The model under review builds one solid part; all positions refer to its coordinate system, in mm. Face numbers are marked on the shaded views. A direction names the side the tool comes from. Give positions to 0.01 mm unless a question says otherwise; leave off trailing zeros. Order: outer loops, then holes, each group sorted by start corner. A loop starts at its lowest first (then second) coordinate and runs counter-clockwise, first axis right, second up.
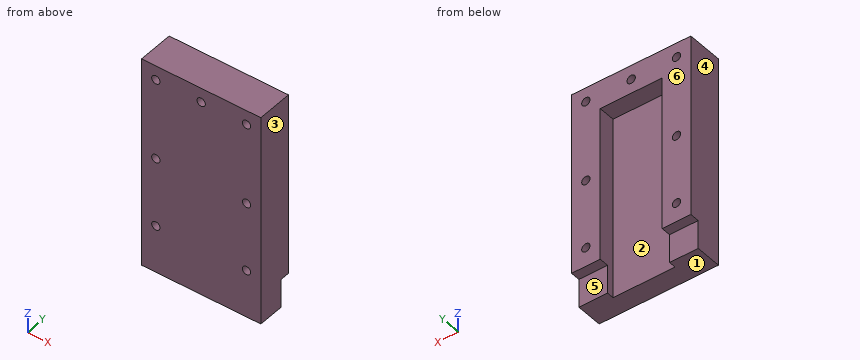
```python
from build123d import *

# Parameters (mm, degrees)
SKETCH_1_W          = 50
SKETCH_1_H          = 30
EXTRUDE_1_DEPTH     = 89
SKETCH_2_W          = 26
SKETCH_2_H          = 14
CUT_EXTRUDE_1_DEPTH = 77
SKETCH_5_W          = 12
SKETCH_5_H          = 8
CUT_EXTRUDE_4_DEPTH = 98.928545379
SKETCH_6_W          = 12
SKETCH_6_H          = 8
CUT_EXTRUDE_5_DEPTH = 98.928545379
SKETCH_7_R          = 1.75
CUT_EXTRUDE_6_DEPTH = 98.190534519


with BuildPart() as part:
    # ｽｹｯﾁ1 → ﾎﾞｽ - 押し出し1 (new body)
    with BuildSketch(Plane.XY):
        Rectangle(SKETCH_1_W, SKETCH_1_H)
    extrude(amount=EXTRUDE_1_DEPTH)

    # ｽｹｯﾁ2 → ｶｯﾄ - 押し出し1 (cut)
    with BuildSketch(Plane(origin=(0, 0, 0), x_dir=(-1, 0, 0), z_dir=(0, 0, -1))):
        Rectangle(SKETCH_2_W, SKETCH_2_H)
    extrude(amount=-CUT_EXTRUDE_1_DEPTH, mode=Mode.SUBTRACT)

    # ｽｹｯﾁ5 → ｶｯﾄ - 押し出し4 (cut, through all)
    with BuildSketch(Plane.ZY.offset(-13)):
        with Locations((6, 0)):
            Rectangle(SKETCH_5_W, SKETCH_5_H)
    extrude(amount=-CUT_EXTRUDE_4_DEPTH, mode=Mode.SUBTRACT)

    # ｽｹｯﾁ6 → ｶｯﾄ - 押し出し5 (cut, through all)
    with BuildSketch(Plane(origin=(-13, 0, 0), x_dir=(0, 0, -1), z_dir=(1, 0, 0))):
        with Locations((-6, 0)):
            Rectangle(SKETCH_6_W, SKETCH_6_H)
    extrude(amount=-CUT_EXTRUDE_5_DEPTH, mode=Mode.SUBTRACT)

    # ｽｹｯﾁ7 → ｶｯﾄ - 押し出し6 (cut, through all)
    with BuildSketch(Plane(origin=(0, 15, 0), x_dir=(1, 0, 0), z_dir=(0, 1, 0))):
        with Locations(Location((19, -20, 0), (0, 0, 270))):
            Circle(SKETCH_7_R)
        with Locations(Location((19, -49, 0), (0, 0, 270))):
            Circle(SKETCH_7_R)
        with Locations(Location((19, -83, 0), (0, 0, 270))):
            Circle(SKETCH_7_R)
        with Locations(Location((0, -83, 0), (0, 0, 270))):
            Circle(SKETCH_7_R)
        with Locations(Location((-19, -83, 0), (0, 0, 270))):
            Circle(SKETCH_7_R)
        with Locations(Location((-19, -49, 0), (0, 0, 270))):
            Circle(SKETCH_7_R)
        with Locations(Location((-19, -20, 0), (0, 0, 270))):
            Circle(SKETCH_7_R)
    extrude(amount=-CUT_EXTRUDE_6_DEPTH, mode=Mode.SUBTRACT)

    # Surface Cut 1
    split(bisect_by=Plane(origin=(0, 0, 0), x_dir=(-1, 0, 0), z_dir=(0, -1, 0)), keep=Keep.TOP)


solid = part.part
```
1. Take a section at C-C (z = 20). Write out the cut boundary in (x, y), and give its area (3 significant figures).
2. Take a section at D-D (z = 83). Write out the cut boundary in (x, y), and give its area (4 significant figures).
3. Insertion check: pin 1 (4 mm diameter, centred on x = 15.5, y = -5.5, fed in from -Z); pin 2 (3 mm diameter, centred on x = 18.5, y = -2, fed in from -Z); pin 3 (3.5 mm diameter, centred on x = -18.5, z = 4, fed in from +Y); pin 4 (3.5 mm diameter, centred on x = -4.5, y = -4.5, fed in from -Z). Each pin has a flat end and moves straight along its axis. Give the tip position at first contact, or say it passes through.
4. To check wall thickness, follow line 1 (X direction, y = -6, z = 49); line 2 (X direction, y = -12, z = 49); line 3 (X direction, y = -7, z = 83). State the ranges of each line that lie inside material, in increasing order.
5. Draft analysis for pull direction X (two halves, no side actions). For the marked faces 1, 2, 3 and 4, state which applies: pulls with the +X half, pulls with the -X half, needs draft (parallel to the pull), parting line crosses it, or undercut.
6. Take a section at B-B (y = -6). Write out the cut boundary in (x, z).
7. For the marked faces 5 and 6, list the 3-axis set-ups (+Z, -Z, +X, -X, +Y, -Y) from which the entire face can be reached by the end or side of a thin tool; tool diameter is ignored.
8. Take a section at A-A (x = 19). Write out the cut boundary in (y, z), and give its area (3 significant figures).
Answer:
1. outline: (-25, -15) - (-20.75, -15) - (-20.75, 0) - (-25, 0) - close; (-17.25, -15) - (17.25, -15) - (17.25, 0) - (13, 0) - (13, -7) - (-13, -7) - (-13, 0) - (-17.25, 0) - close; (20.75, -15) - (25, -15) - (25, 0) - (20.75, 0) - close
1. area: 463 mm2
2. outline: (-25, -15) - (-20.75, -15) - (-20.75, 0) - (-25, 0) - close; (-17.25, -15) - (-1.75, -15) - (-1.75, 0) - (-17.25, 0) - close; (1.75, -15) - (17.25, -15) - (17.25, 0) - (1.75, 0) - close; (20.75, -15) - (25, -15) - (25, 0) - (20.75, 0) - close
2. area: 592.5 mm2
3. pin 1: stops at z = 0
3. pin 2: stops at z = 12
3. pin 3: stops at y = -4
3. pin 4: stops at z = 77
4. line 1: x = -25 to -20.75, -17.25 to -13, 13 to 17.25, 20.75 to 25
4. line 2: x = -25 to -20.75, -17.25 to 17.25, 20.75 to 25
4. line 3: x = -25 to -20.75, -17.25 to -1.75, 1.75 to 17.25, 20.75 to 25
5. face 1: needs draft
5. face 2: undercut
5. face 3: pulls with the +X half
5. face 4: pulls with the -X half
6. outline: (-25, 0) - (-13, 0) - (-13, 77) - (13, 77) - (13, 0) - (25, 0) - (25, 89) - (-25, 89) - close; hole circle Ø3.5 at (-19, 20); hole circle Ø3.5 at (-19, 49); hole circle Ø3.5 at (-19, 83); hole circle Ø3.5 at (0, 83); hole circle Ø3.5 at (19, 20); hole circle Ø3.5 at (19, 49); hole circle Ø3.5 at (19, 83)
7. face 5: -Z, +X, -X, +Y
7. face 6: +Z, -Z, +X, -X, +Y
8. outline: (-15, 0) - (-4, 0) - (-4, 12) - (0, 12) - (0, 18.25) - (-15, 18.25) - close; (-15, 21.75) - (0, 21.75) - (0, 47.25) - (-15, 47.25) - close; (-15, 50.75) - (0, 50.75) - (0, 81.25) - (-15, 81.25) - close; (-15, 84.75) - (0, 84.75) - (0, 89) - (-15, 89) - close
8. area: 1,130 mm2
